```python
from build123d import *

# Parameters (mm, degrees)
F1_DEPTH = 50.8
F3_DEPTH = 6.35
F5_DEPTH = 6.35


with BuildPart() as f1:
    # F0 (on Front) → F1 (new body, symmetric)
    with BuildSketch(Plane.XZ):
        Polygon((-50.8, 12.817732), (-50.8, -13.73706), (50.8, -13.73706), (50.8, 12.817732), (45.72, 12.817732), (45.72, -8.65706), (-45.72, -8.65706), (-45.72, 12.817732), align=None)
    extrude(amount=F1_DEPTH, both=True)

    # F2 (on face) → F3 (join)
    with BuildSketch(Plane(origin=(0, 50.8, 0), x_dir=(-1, 0, 0), z_dir=(0, 1, 0))):
        Polygon((45.72, 12.817732), (50.8, 12.817732), (12.7, 50.917732), (12.7, 76.317732), (-12.7, 76.317732), (-12.7, 50.917732), (-50.8, 12.817732), (-45.72, 12.817732), (-45.72, -8.65706), (45.72, -8.65706), align=None)
    extrude(amount=-F3_DEPTH)

    # F4 (on face) → F5 (cut, through all)
    with BuildSketch(Plane(origin=(0, 50.8, 0), x_dir=(-1, 0, 0), z_dir=(0, 1, 0))):
        Polygon((-31.75, -8.65706), (31.75, -8.65706), (31.75, 10.392591), (-31.865364, 10.392591), align=None)
    extrude(amount=-F5_DEPTH, mode=Mode.SUBTRACT)


solid = f1.part
```
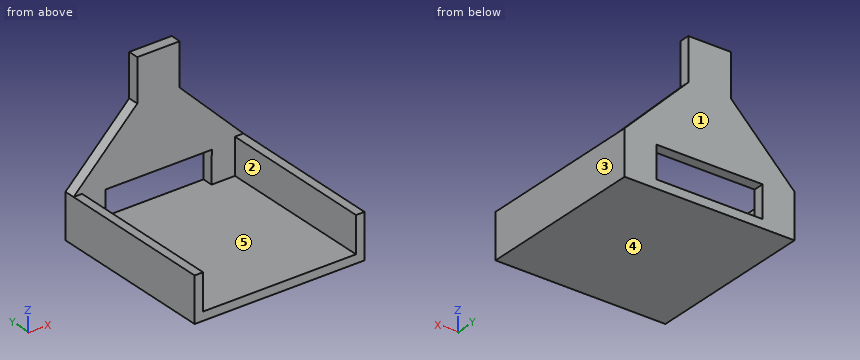
Here's how the part is built. I have some questions about the finished solid (model axes, mm). Face numbers are marked on the shaded views. A direction names the side the tool comes from. Round coordinates to 2 decimals unless told otherwise and drop trailing zeros. Write each loop counter-clockwise with the first axis right and the second up, starting at its lowest first coordinate (ties: lowest second). Pieces come first, ordered by that corner, then holes.
Q1. If we section it at A-A on x = 1.5: Write out the boundary of the cut face in (y, z).
Q2. Will these pins go through, and if not, where does the flat tip stop? P1, Ø5.5, axis at x = -49.5, y = 6.5, coming from the +Z side; P2, Ø1.5, axis at x = -27, y = 6.5, coming from the +Z side; P3, Ø3, axis at y = 46.5, z = 68.5, coming from the +X side.
Q3. Which directions (+Z, -Z, +X, -X, +Y, -Y) give clear straight access to the entire face, cutting with the end or side of a thin tool? Please do the marked faces 1 and 2.
Q4. If we section it at C-C on y = -19.5: Write out the boundary of the cut face in (x, z), plus the area to 3 significant figures.
Q5. Please list where these lines run through material, in increasing order: probe 1 along X at (y, z) = (2, 6); probe 2 along Z at (x, y) = (-21, -20); probe 3 along Y at (x, z) = (7, 11.5).
Q6. If we section it at D-D on z = 67: Write out the boundary of the cut face in (x, y).
Q7. If we mould it in two halves opening along X, with no side actions, what happens to the marked faces 3, 4 and 5? For each: +X half, -X half, draft (parallel to the pull), parting line (faces both ways), or undercut.
Q8. If we section it at B-B on z = 7: Write out the boundary of the cut face in (x, y), plus the area to 3 significant figures.
Answer below:
1. outline: (-50.8, -13.74) - (50.8, -13.74) - (50.8, -8.66) - (-50.8, -8.66) - close; (44.45, 10.39) - (50.8, 10.39) - (50.8, 76.32) - (44.45, 76.32) - close
2. P1: stops at z = 12.82
2. P2: stops at z = -8.66
2. P3: stops at x = 12.7
3. face 1: +Z, -Z, +X, -X, +Y
3. face 2: +Z, -Y
4. outline: (-50.8, -13.74) - (50.8, -13.74) - (50.8, 12.82) - (45.72, 12.82) - (45.72, -8.66) - (-45.72, -8.66) - (-45.72, 12.82) - (-50.8, 12.82) - close
4. area: 734 mm2
5. probe 1: x = -50.8 to -45.72, 45.72 to 50.8
5. probe 2: z = -13.74 to -8.66
5. probe 3: y = 44.45 to 50.8
6. outline: (-12.7, 44.45) - (12.7, 44.45) - (12.7, 50.8) - (-12.7, 50.8) - close
7. face 3: +X half
7. face 4: draft
7. face 5: undercut
8. outline: (-50.8, -50.8) - (-45.72, -50.8) - (-45.72, 44.45) - (-31.75, 44.45) - (-31.75, 50.8) - (-50.8, 50.8) - close; (31.84, 44.45) - (45.72, 44.45) - (45.72, -50.8) - (50.8, -50.8) - (50.8, 50.8) - (31.84, 50.8) - close
8. area: 1,210 mm2
